The model under review builds one solid part; all positions refer to its coordinate system, in mm. A direction names the side the tool comes from. Give positions to 0.01 mm unless a question says otherwise; leave off trailing zeros. Loops run counter-clockwise (first coordinate to the right, second up) from the corner with the lowest first, then second, coordinate; pieces in that order, holes last. Notation, with made-up numbers: (53.25, 12) - (61.25, 12) arc R29 cw to (61.25, 51) - close; hole circle Ø7 at (-31, -39). An arc over 180 degrees is marked (long way). Return JSON: item names as keys, results as strings. Group by question number.
from build123d import *

# Parameters (mm, degrees)
SKETCH1_R           = 1.27
BOSS_EXTRUDE1_DEPTH = 3.175


with BuildPart() as part:
    # Sketch1 → Boss-Extrude1 (new body)
    with BuildSketch(Plane(origin=(0, 0, 0), x_dir=(1, 0, 0), z_dir=(0, 1, 0))):
        Polygon((27.49630657, 15.875), (0, 31.75), (-27.49630657, 15.875), (-27.49630657, -15.875), (0, -31.75), (27.49630657, -15.875), align=None)
        with Locations(Location((0, 0, 0), (0, 0, 270))):
            Circle(SKETCH1_R, mode=Mode.SUBTRACT)
        Polygon((-13.422443502, 20.276025186), (-11.234134179, 21.565560882), (-8.01029494, 16.094787576), (-10.198604263, 14.805251881), align=None, mode=Mode.SUBTRACT)
        Polygon((7.722422107, 16.234876315), (10.848331148, 21.762189646), (13.059256481, 20.51182603), (9.933347439, 14.984512698), align=None, mode=Mode.SUBTRACT)
        Polygon((17.921026369, 1.429624434), (24.27077465, 1.48616446), (24.29339066, -1.053734852), (17.94364238, -1.110274878), align=None, mode=Mode.SUBTRACT)
        Polygon((10.198604263, -14.805251881), (13.422443502, -20.276025186), (11.234134179, -21.565560882), (8.01029494, -16.094787576), align=None, mode=Mode.SUBTRACT)
        Polygon((-7.722422107, -16.234876315), (-10.848331148, -21.762189646), (-13.059256481, -20.51182603), (-9.933347439, -14.984512698), align=None, mode=Mode.SUBTRACT)
        Polygon((-17.921026369, -1.429624434), (-24.27077465, -1.48616446), (-24.29339066, 1.053734852), (-17.94364238, 1.110274878), align=None, mode=Mode.SUBTRACT)
    extrude(amount=-BOSS_EXTRUDE1_DEPTH)


solid = part.part
Item 1: For L1, parallel to X at y = -2.45, z = 0; L2, parallel to X at y = -1.2, z = 20; L3, parallel to X at y = -2.85, z = 16, list the stretches that pass through material, from the lowest coordinate up. Write a range as from..to.
Item 2: Take a section at D-D (z = -18). State the section outline as (x, y) points (3 decimals), then the cut area to 3 significant figures.
Item 3: Take a section at C-C (y = -2.45). State how many separate pieces and enclosed holes the cut face has, then the cut area to 3 significant figures.
Item 4: Tool access review of faces 1 (the face through (-9.645, -1.565, -18.868)), 2 (the face through (-6, -3.175, 0)): name each direction out of +Z, -Z, +X, -X, +Y, -Y from which nothing blocks a thin tool from reaching the whole face with its end or side.
Item 5: For P1, Ø2, axis at x = 0, z = 0, coming from the -Y side; P2, Ø1, axis at x = 9.5, y = -0.5, coming from the +Z side, all flat-tipped, find the tip position at first contact; note any pin that passes through.
Item 6: Mouldability with a two-part tool opening along Z and no side actions: class faces 3 (the face through (-11.938, -1.565, 21.146)), 4 (the face through (-13.6, -1.6, -23.9)), 5 (the face through (-27.496, -2, 0)), 6 (the face through (-13.94, -1.57, 23.7)) as +Z half, -Z half, draft (parallel to the pull), parting line (faces both ways), or undercut.
Item 7: Take a section at B-B (z = 0). State the section outline as (x, y) points (3 decimals), then the cut area to 3 significant figures.
Item 8: Take a section at A-A (x = -22.5). State the section outline as (y, z) points (3 decimals).
Check sheet entries:
{
 "1": {"L1": "x = -27.5..-24.28, -17.93..-1.27, 1.27..17.93, 24.28..27.5", "L2": "x = -20.35..-12.77, -9.85..10.31, 13.26..20.35", "L3": "x = -27.28..-10.51, -8.14..8.17, 10.9..27.28"},
 "2": {"outline": "(-23.816, -3.175) - (-12.081, -3.175) - (-12.081, 0) - (-23.816, 0) - close; (-9.133, -3.175) - (8.721, -3.175) - (8.721, 0) - (-9.133, 0) - close; (11.639, -3.175) - (23.816, -3.175) - (23.816, 0) - (11.639, 0) - close", "area": "133 mm^2"},
 "3": {"separate pieces": "1", "enclosed holes": "7", "area": "2,520 mm^2"},
 "4": {"face 1": "+Y, -Y", "face 2": "+Z, -Z, +X, -X, -Y"},
 "5": {"P1": "passes through", "P2": "stops at z = 26.55"},
 "6": {"face 3": "undercut", "face 4": "-Z half", "face 5": "draft", "face 6": "+Z half"},
 "7": {"outline": "(-27.496, -3.175) - (-24.284, -3.175) - (-24.284, 0) - (-27.496, 0) - close; (-17.934, -3.175) - (-1.27, -3.175) - (-1.27, 0) - (-17.934, 0) - close; (1.27, -3.175) - (17.934, -3.175) - (17.934, 0) - (1.27, 0) - close; (24.284, -3.175) - (27.496, -3.175) - (27.496, 0) - (24.284, 0) - close", "area": "126 mm^2"},
 "8": {"outline": "(-3.175, -18.76) - (0, -18.76) - (0, -1.07) - (-3.175, -1.07) - close; (-3.175, 1.47) - (0, 1.47) - (0, 18.76) - (-3.175, 18.76) - close"}
}
